Geometry check sheet. Reference: the model listing, model coordinates, mm. Round coordinates to 2 decimals unless told otherwise and drop trailing zeros. Write each loop counter-clockwise with the first axis right and the second up, starting at its lowest first coordinate (ties: lowest second). Pieces come first, ordered by that corner, then holes.
Autodesk Fusion 360 part; units mm, degrees
sketch "Esquisse1" plane through (0, 0, 0) normal (0, 0, 1) x (1, 0, 0)
  line L0 (0, 0) -> (59, 0)
  line L1 (59, 0) -> (59, 22)
  line L2 (59, 22) -> (0, 22)
  line L3 (0, 22) -> (0, 0)
  line L4 (0, 0) -> (0, 17) construction
  line L5 (0, 17) -> (0, 39) construction
  arc A0 (0, 17) -> (13.9642, 22) centre (0, 39) ccw
  dimension "d1" = 22
  dimension "d2" = 59
  dimension "d3" = 17
  dimension "d4" = 22
extrude "Extrusion1" add sketch "Esquisse1" along normal blind 2 contours L0 L1 L2 L3 A0
sketch "Esquisse2" plane through (0, 0, 2) normal (0, 0, 1) x (-1, 0, 0)
  line L0 (0, 0) -> (-59, 0)
  line L1 (-59, 0) -> (-59, -22)
  line L2 (-59, -22) -> (-13.9642, -22)
  arc A0 (0, -17) -> (-13.9642, -22) centre (0, -39) ccw
  line L3 (0, -17) -> (0, 0)
  arc A1 (-1.4, -15.6419) -> (-14.4568, -20.6) centre (0, -39) ccw
  line L4 (-57.6, -20.6) -> (-14.4568, -20.6)
  line L5 (-57.6, -1.4) -> (-57.6, -20.6)
  line L6 (-1.4, -1.4) -> (-57.6, -1.4)
  line L7 (-1.4, -15.6419) -> (-1.4, -1.4)
  dimension "d7" = -1.4
extrude "Extrusion11" add sketch "Esquisse2" against normal blind 3.7 contours A1 L4 L5 L6 L7
chamfer "Chanfrein3" distance 0.3 angle 45 5 edges at (29.5, 1.4, -1.7) (1.4, 8.521, -1.7) (8.307, 17.1241, -1.7) (36.0284, 20.6, -1.7) (57.6, 11, -1.7)
fillet "Congé7" radius 1.5 3 edges at (0, 0, 1) (59, 0, 1) (59, 22, 1)
fillet "Congé8" radius 1 2 edges at (13.9642, 22, 1) (0, 17, 1)
fillet "Congé9" radius 0.5 10 edges at (0.4393, 0.4393, 2) (29.5, 0, 2) (58.5607, 0.4393, 2) (59, 11, 2) (58.5607, 21.5607, 2) (35.9089, 22, 2) (13.9881, 21.9441, 2) (7.7031, 18.3927, 2) (0.2777, 16.7133, 2) (0, 8.7609, 2)
hole "Perçage1" at (43.74, 11, 2) direction (0, 0, -1) diameter 1.5 depth 9 tip angle 180 counterbore diameter 3 counterbore depth 2
pattern_linear "Réseau R1" count 2 spacing 30 along (-1, 0, 0) of "Perçage1"
equation "d76 = d5"
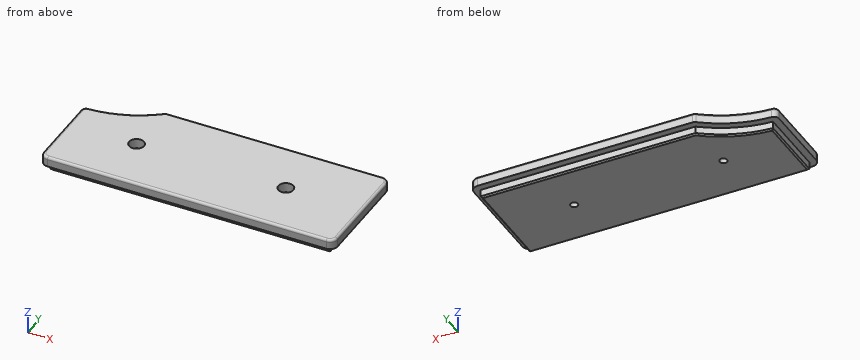
1. Section check B-B (y = 11). Record the cut outline in (x, z), plus the area to 3 significant figures.
2. Section check C-C (z = 0.75). Record the cut outline in (x, y).
3. Depth check by flat-ended pin: pin 1 Ø1.1 at (y, z) = (14, -1) entering from +X; pin 2 Ø1.7 at (x, y) = (43.74, 11) entering from +Z; pin 3 Ø1.5 at (x, z) = (25.5, -1) entering from -Y. Enter the tip coordinate at first touch or a pass-through.
4. Scan lines: line 1 along X through (y, z) = (11, 1.6); line 2 along X through (y, z) = (11, -1.3); line 3 along Y through (x, z) = (43.74, -0.95). Record each from-to range of solid material in increasing order.
5. Section check D-D (y = 2.25). Record the cut outline in (x, z), plus the area to 3 significant figures.
6. Section check A-A (x = 43.74). Record the cut outline in (y, z), plus the area to 3 significant figures.
Results below:
1. outline: (0, 0) - (1.4, 0) - (1.4, -1.4) - (1.7, -1.7) - (12.99, -1.7) - (12.99, 0) - (12.24, 0) - (12.24, 2) - (0.5, 2) arc R0.5 ccw to (0, 1.5) - close; (14.49, -1.7) - (42.99, -1.7) - (42.99, 0) - (42.24, 0) - (42.24, 2) - (15.24, 2) - (15.24, 0) - (14.49, 0) - close; (44.49, -1.7) - (57.3, -1.7) - (57.6, -1.4) - (57.6, 0) - (59, 0) - (59, 1.5) arc R0.5 ccw to (58.5, 2) - (45.24, 2) - (45.24, 0) - (44.49, 0) - close
1. area: 196 mm2
2. outline: (0, 1.5) arc R1.5 ccw to (1.5, 0) - (57.5, 0) arc R1.5 ccw to (59, 1.5) - (59, 20.5) arc R1.5 ccw to (57.5, 22) - (14.32, 22) arc R1 ccw to (13.7, 21.78) arc R22 cw to (0.96, 17.02) arc R1 ccw to (0, 16.02) - close; hole circle Ø3 at (13.74, 11); hole circle Ø3 at (43.74, 11)
3. pin 1: stops at x = 57.6
3. pin 2: stops at z = 0
3. pin 3: stops at y = 1.4
4. line 1: x = 0.01 to 12.24, 15.24 to 42.24, 45.24 to 58.99
4. line 2: x = 1.4 to 12.99, 14.49 to 42.99, 44.49 to 57.6
4. line 3: y = 1.4 to 10.25, 11.75 to 20.6
5. outline: (0, 0) - (1.4, 0) - (1.4, -1.4) - (1.7, -1.7) - (57.3, -1.7) - (57.6, -1.4) - (57.6, 0) - (59, 0) - (59, 1.5) arc R0.5 ccw to (58.5, 2) - (0.5, 2) arc R0.5 ccw to (0, 1.5) - close
5. area: 213 mm2
6. outline: (0, 0) - (1.4, 0) - (1.4, -1.4) - (1.7, -1.7) - (10.25, -1.7) - (10.25, 0) - (9.5, 0) - (9.5, 2) - (0.5, 2) arc R0.5 ccw to (0, 1.5) - close; (11.75, -1.7) - (20.3, -1.7) - (20.6, -1.4) - (20.6, 0) - (22, 0) - (22, 1.5) arc R0.5 ccw to (21.5, 2) - (12.5, 2) - (12.5, 0) - (11.75, 0) - close
6. area: 67.9 mm2
